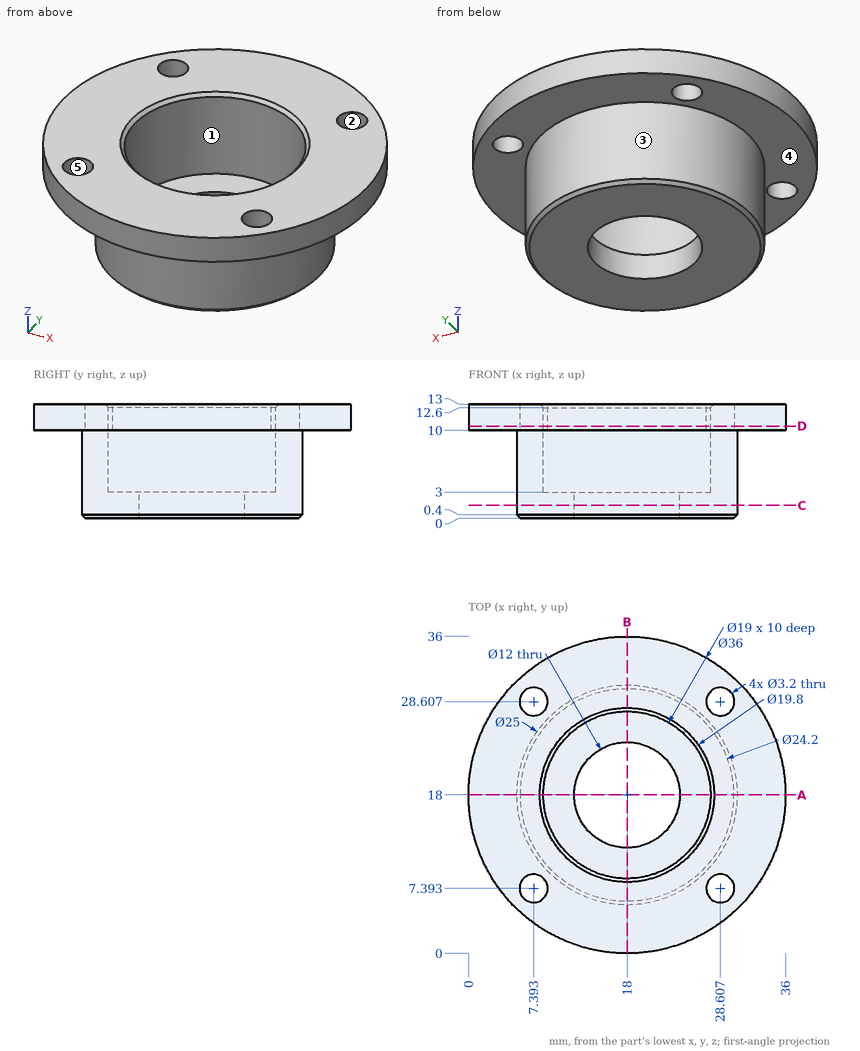
Drawing for the job (mm, zero at the part's lowest x, y, z). A direction names the side the tool comes from. Round coordinates to 2 decimals unless told otherwise and drop trailing zeros. Order: outer loops, then holes, each group sorted by start corner. A loop starts at its lowest first (then second) coordinate and runs counter-clockwise, first axis right, second up.
Item 1: Saw through at D-D on z = 10.5. Write the cut outline in (x, y).
Item 2: Saw through at A-A on y = 18. Write the cut outline in (x, z).
Item 3: Saw through at C-C on z = 1.5. Write the cut outline in (x, y).
Item 4: Pin check, flat tips, straight feed: pin 1 (3.5 mm diameter, centred on x = 7.39, y = 28.61, fed in from -Z); pin 2 (1.5 mm diameter, centred on x = 12, z = 5, fed in from -Y) (1 decimal); pin 3 (1.9 mm diameter, centred on x = 28.61, y = 7.39, fed in from -Z); pin 4 (3 mm diameter, centred on x = 16.5, z = 11, fed in from -Y). Stop position of each tip, or through.
Item 5: Tool access for the marked faces 1 and 2: list every direction of +Z, -Z, +X, -X, +Y, -Y with a clear straight run to the whole face (end or side of a thin tool).
Item 6: Mould opens along Y. For the marked faces 3, 4 and 5 say: pulls with the +Y half, pulls with the -Y half, needs draft (parallel to the pull), parting line crosses it, or undercut.
Item 7: Probe line 1 along Y through (x, z) = (18, 1.95); line 2 along Y through (x, z) = (18, 3.25); line 3 along Z through (x, y) = (23, 32). List the from-to ranges inside material, lowest first.
Reported:
1. outline: circle Ø36 at (18, 18); hole circle Ø3.2 at (7.39, 7.39); hole circle Ø3.2 at (7.39, 28.61); hole circle Ø19 at (18, 18); hole circle Ø3.2 at (28.61, 7.39); hole circle Ø3.2 at (28.61, 28.61)
2. outline: (0, 10) - (5.5, 10) - (5.5, 0.4) - (5.9, 0) - (12, 0) - (12, 3) - (8.5, 3) - (8.5, 12.6) - (8.1, 13) - (0, 13) - close; (24, 0) - (30.1, 0) - (30.5, 0.4) - (30.5, 10) - (36, 10) - (36, 13) - (27.9, 13) - (27.5, 12.6) - (27.5, 3) - (24, 3) - close
3. outline: circle Ø25 at (18, 18); hole circle Ø12 at (18, 18)
4. pin 1: stops at z = 10
4. pin 2: stops at y = 6.7
4. pin 3: passes through
4. pin 4: stops at y = 0
5. face 1: +Z
5. face 2: +Z, -Z
6. face 3: parting line crosses it
6. face 4: needs draft
6. face 5: undercut
7. line 1: y = 5.5 to 12, 24 to 30.5
7. line 2: y = 5.5 to 8.5, 27.5 to 30.5
7. line 3: z = 10 to 13
